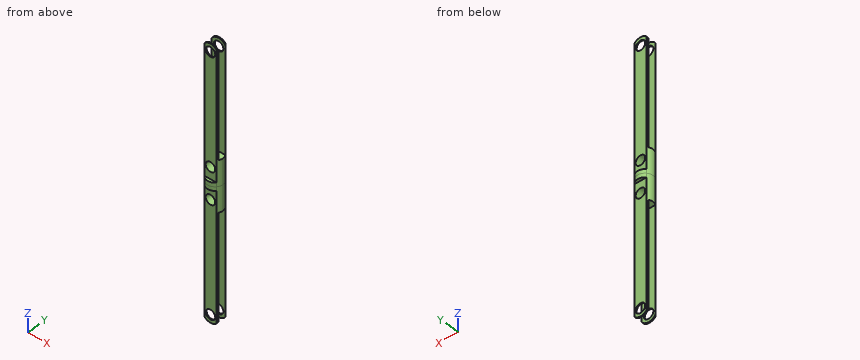
```python
from build123d import *

# Parameters (mm, degrees)
EXTRUDE_1_DEPTH          = 100
CUT_EXTRUDE_START        = -1.6
CUT_EXTRUDE_2_OUTLINE_W  = 11.543856376
CUT_EXTRUDE_2_OUTLINE_H  = 103.894707388
CUT_EXTRUDE_2_OUTLINE_R  = 1.5
CUT_EXTRUDE_2_DEPTH      = 3.2
CUT_EXTRUDE_3_DEPTH      = 22
CUT_EXTRUDE_3_DEPTH_BACK = 22
SKETCH_6_W               = 64
SKETCH_6_H               = 2.5
EXTRUDE_START            = -1.25
SKETCH_7_R               = 2.5
EXTRUDE_2_DEPTH          = 1.25


# Read off the part's stored shape, not the designer's step: 切除-拉伸2
with BuildPart() as part:
    # 草图1 → 凸台-拉伸1 (new body)
    with BuildSketch(Plane.XY):
        with BuildLine():
            Line((1.920937271, 1.6), (0, 1.6))
            Line((0, 1.6), (0, -1.6))
            Line((0, -1.6), (1.920937271, -1.6))
            ThreePointArc((1.920937271, -1.6), (2.350781059, -0.850781059), (2.5, 0))
            ThreePointArc((2.5, 0), (2.350781059, 0.850781059), (1.920937271, 1.6))
        make_face()
        with BuildLine():
            Line((0, -1.6), (0, 1.6))
            Line((0, 1.6), (-1.920937271, 1.6))
            ThreePointArc((-1.920937271, 1.6), (-2.5, 0), (-1.920937271, -1.6))
            Line((-1.920937271, -1.6), (0, -1.6))
        make_face()
    extrude(amount=EXTRUDE_1_DEPTH)

    # 切除-拉伸2 outline → 切除-拉伸2 (cut)
    # profile 1 of 3: a face of its own
    with BuildSketch(Plane(origin=(0, 0, 0), x_dir=(1, 0, 0), z_dir=(0, 1, 0)).offset(CUT_EXTRUDE_START)):
        with Locations((0.333099219, -49.873134062)):
            Rectangle(CUT_EXTRUDE_2_OUTLINE_W, CUT_EXTRUDE_2_OUTLINE_H)
        with BuildLine():
            Line((-2.5, -50), (-2.5, -10))
            ThreePointArc((-2.5, -10), (0, -7.5), (2.5, -10))
            Line((2.5, -10), (2.5, -50))
            Line((2.5, -50), (-2.5, -50))
        make_face(mode=Mode.SUBTRACT)
    # profile 2 of 3: a face of its own
    with BuildSketch(Plane(origin=(0, 0, 0), x_dir=(1, 0, 0), z_dir=(0, 1, 0)).offset(CUT_EXTRUDE_START)):
        with Locations((0, -45)):
            Circle(CUT_EXTRUDE_2_OUTLINE_R)
    # profile 3 of 3: a face of its own
    with BuildSketch(Plane(origin=(0, 0, 0), x_dir=(1, 0, 0), z_dir=(0, 1, 0)).offset(CUT_EXTRUDE_START)):
        with Locations((0, -10)):
            Circle(CUT_EXTRUDE_2_OUTLINE_R)
    extrude(amount=CUT_EXTRUDE_2_DEPTH, mode=Mode.SUBTRACT)

    # 草图6 → 切除-拉伸3 (cut, two sides: drawn at the far end of the back side and taken through both)
    with BuildSketch(Plane(origin=(0, 0, 0), x_dir=(0, 0, -1), z_dir=(1, 0, 0)).offset(-CUT_EXTRUDE_3_DEPTH_BACK)):
        with Locations((-10, 0)):
            Rectangle(SKETCH_6_W, SKETCH_6_H)
    extrude(amount=CUT_EXTRUDE_3_DEPTH + CUT_EXTRUDE_3_DEPTH_BACK, mode=Mode.SUBTRACT)

    # 草图7 → 凸台-拉伸2 (add)
    with BuildSketch(Plane.XY.offset(50).offset(EXTRUDE_START)):
        with Locations(Location((0, 0, 0), (0, 0, 150))):
            Circle(SKETCH_7_R)
    extrude(amount=EXTRUDE_2_DEPTH)

    # 镜向1: part across face


with BuildPart() as part_1:
    add(part.part)
    add(part.part.mirror(Plane.XY.offset(50)))


solid = part_1.part
```
Could you check a few things on this model? Use its own coordinates, in mm. Give positions to 0.01 mm unless a question says otherwise; leave off trailing zeros. Loops run counter-clockwise (first coordinate to the right, second up) from the corner with the lowest first, then second, coordinate; pieces in that order, holes last. Notation, with made-up numbers: (38, 70) - (47, 70) arc R20 ccw to (47, 95) - close; hole circle Ø2 at (-25, 89). An arc over 180 degrees is marked (long way). Answer in a Markdown table with one row per item. Add a question column.
Q1. If we section it at B-B (z = 90): List the corners of the cut face in (x, y) for me.
Q2. If we section it at C-C (x = 0): State how many separate pieces and enclosed holes the cut face has, plus the area to 3 significant figures.
Q3. If we section it at A-A (z = 28): List the corners of the cut face in (x, y) for me.
Q4. For pin 1 (1.2 mm diameter, centred on x = 1, z = 38, fed in from -Y); pin 2 (1.2 mm diameter, centred on x = -0.5, z = 77.5, fed in from +Y); pin 3 (2.5 mm diameter, centred on x = 0, z = 90, fed in from -Y); pin 4 (1 mm diameter, centred on x = -0.5, y = 1.5, fed in from +Z), each with a flat end and sliding along its axis, tell me the tip position at first contact or that it passes through.
Q5. If we section it at D-D (z = 55): List the corners of the cut face in (x, y) for me, plus the area to 3 significant figures.
Q6. Please list where these lines run through material, in increasing order: L1, parallel to Z at x = 0, y = -1.4; L2, parallel to Z at x = 0, y = 0.2; L3, parallel to Y at x = 1.8, z = 76.5. Write a range as from..to.
The answers:
| question | item | result |
|---|---|---|
| 1 | outline | (-2.17, -1.25) arc R2.5 ccw to (-1.92, -1.6) - (-1.5, -1.6) - (-1.5, -1.25) - close; (-2.17, 1.25) - (-1.5, 1.25) - (-1.5, 1.6) - (-1.92, 1.6) arc R2.5 ccw to start; (1.5, -1.6) - (1.92, -1.6) arc R2.5 ccw to (2.17, -1.25) - (1.5, -1.25) - close; (1.5, 1.25) - (2.17, 1.25) arc R2.5 ccw to (1.92, 1.6) - (1.5, 1.6) - close |
| 2 | separate pieces | 7 |
| 2 | enclosed holes | 0 |
| 2 | area | 80.6 mm^2 |
| 3 | outline | (-2.17, -1.25) arc R2.5 ccw to (-1.92, -1.6) - (1.92, -1.6) arc R2.5 ccw to (2.17, -1.25) - close; (-2.17, 1.25) - (2.17, 1.25) arc R2.5 ccw to (1.92, 1.6) - (-1.92, 1.6) arc R2.5 ccw to start |
| 4 | pin 1 | stops at y = -1.6 |
| 4 | pin 2 | stops at y = 1.6 |
| 4 | pin 3 | passes through |
| 4 | pin 4 | stops at z = 92.5 |
| 5 | outline | (-1.92, -1.6) - (-1.5, -1.6) - (-1.5, 1.6) - (-1.92, 1.6) arc R2.5 ccw to start; (1.5, -1.6) - (1.92, -1.6) arc R2.5 ccw to (1.92, 1.6) - (1.5, 1.6) - close |
| 5 | area | 5.23 mm^2 |
| 6 | L1 | z = 7.5..8.5, 11.5..43.5, 46.5..53.5, 56.5..88.5, 91.5..92.5 |
| 6 | L2 | z = 42..43.5, 46.5..53.5, 56.5..58 |
| 6 | L3 | y = -1.6..-1.25, 1.25..1.6 |
